Here's how the part is built. I have some questions about the finished solid (model axes, mm). Face numbers are marked on the shaded views. A direction names the side the tool comes from. Round coordinates to 2 decimals unless told otherwise and drop trailing zeros. Order: outer loops, then holes, each group sorted by start corner. A loop starts at its lowest first (then second) coordinate and runs counter-clockwise, first axis right, second up. Notation, with made-up numbers: M -8.75,77.5 L -4.75,77.5 A26 cw -4.75,112.5 Z; hole C -17.5,56 d1. An arc over 180 degrees is marked long. Write item = value, one per line. Start each with the question number.
Item 1: I want a section at B-B, the plane y = 0. List the corners of the cut face in (x, z) for me.
Item 2: For the marked faces 1, 2 and 3, which set-ups out of +Z, -Z, +X, -X, +Y, -Y let a thin tool reach every point of the face, with its end or its side?
Item 3: I'm going to push flat-ended pins straight in: P1, Ø6, axis at y = 14.5, z = 5, coming from the +X side; P2, Ø2, axis at x = -2, z = 4.5, coming from the +Y side; P3, Ø1, axis at x = -13, y = -31.5, coming from the -Z side. Where does each tip first touch, or does it pass through?
Item 4: Please list where these lines run through material, in increasing order: L1, parallel to Z at x = 10, y = 11; L2, parallel to Y at x = -7.5, z = 3.5; L3, parallel to Y at x = 0, z = -1.6.
Item 5: I want a section at A-A, the plane x = 0. List the corners of the cut face in (y, z) for me.
Item 6: We'd pull the mould along X, two halves only. Please class the marked faces 4, 5 and 6: pulls with the +X half, pulls with the -X half, needs draft (parallel to the pull), parting line crosses it, or undercut.
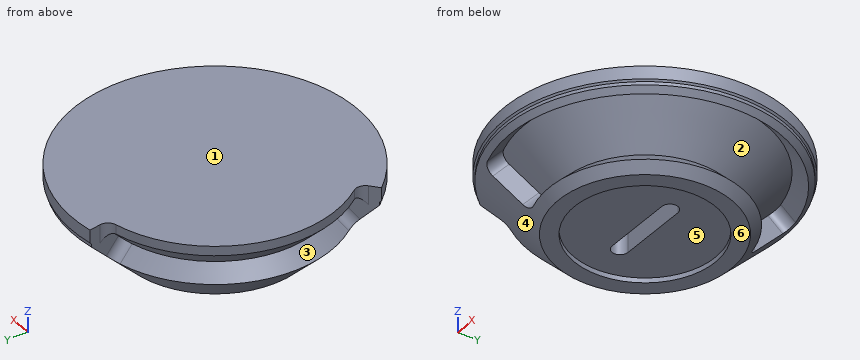
```python
from build123d import *

# Parameters (mm, degrees)
F3_W           = 8.3933982822
F3_H           = 16.3933982822
F4_ANGLE_BACK  = 40
F4_ANGLE       = 122
F6_ANGLE_START = 98
F6_ANGLE       = 196
F7_ANGLE_BACK  = 40
F7_ANGLE       = 122
F8_R           = 3
F8_2_R         = 3
F9_R           = 3
F13_DEPTH      = 10
F14_R          = 22
F15_DEPTH      = 1.5


with BuildPart() as f1:
    # F0 (on Front) → F1 (revolve)
    with BuildSketch(Plane.XZ):
        Polygon((-43.5, 14.5), (-27, -2), (0, -2), (0, 20), (-44, 20), (-44, 16), (-43.5, 15.5), align=None)
    revolve(axis=Axis((0, 0, 9.4880101401), (0, 0, -1)))


with BuildPart() as f4:
    # F3 (on Front) → F4 (revolve)
    with BuildSketch(Plane.XZ, mode=Mode.PRIVATE) as f4_sk:
        with Locations((-41.8033008589, 16.8033008589)):
            Rectangle(F3_W, F3_H)
    revolve(f4_sk.sketch.rotate(Axis((0, 0, 9.4880101401), (0, 0, -1)), -F4_ANGLE_BACK), axis=Axis((0, 0, 9.4880101401), (0, 0, -1)), revolution_arc=F4_ANGLE)

    # F8#2
    f8_2_edges = [f4.edges().sort_by_distance(p)[0] for p in [
        (-5.233827, 37.240617, 16.803301),
        (-28.808328, -24.173058, 16.803301),
    ]]
    fillet(f8_2_edges, radius=F8_2_R)


with BuildPart() as f6:
    # F5 (on Front) → F6 (revolve)
    with BuildSketch(Plane.XZ, mode=Mode.PRIVATE) as f6_sk:
        Polygon((-36.8994949366, -6.2426406871), (-25.5857864376, 5.0710678119), (-37.6066017178, 17.091883092), (-48.9203102168, 5.7781745931), align=None)
    revolve(f6_sk.sketch.rotate(Axis((0, 0, 9), (0, 0, -1)), F6_ANGLE_START), axis=Axis((0, 0, 9), (0, 0, -1)), revolution_arc=F6_ANGLE)

    # F9
    f9_edges = [f6.edges().sort_by_distance(p)[0] for p in [
        (4.348135, 30.938589, -0.585786),
        (6.021109, 42.842419, 11.435029),
        (-17.596833, -39.523134, 11.435029),
        (-12.707527, -28.541572, -0.585786),
    ]]
    fillet(f9_edges, radius=F9_R)


with BuildPart() as f7:
    # F2 (on Front) → F7 (revolve)
    with BuildSketch(Plane.XZ, mode=Mode.PRIVATE) as f7_sk:
        Polygon((-41.2877159425, 2.0970603683), (-31.9497474683, 11.4350288425), (-37.6066017178, 17.091883092), (-46.944570192, 7.7539146178), align=None)
    revolve(f7_sk.sketch.rotate(Axis((0, 0, 9), (0, 0, -1)), -F7_ANGLE_BACK), axis=Axis((0, 0, 9), (0, 0, -1)), revolution_arc=F7_ANGLE)

    # F8
    f8_edges = [f7.edges().sort_by_distance(p)[0] for p in [
        (-28.051576, -23.538067, 6.766045),
        (-5.096342, 36.262361, 6.766045),
    ]]
    fillet(f8_edges, radius=F8_R)


with BuildPart() as f1_1:
    add(f1.part)

    # F10: cut F7, F4, F6
    add(f7.part, mode=Mode.SUBTRACT)
    add(f4.part, mode=Mode.SUBTRACT)
    add(f6.part, mode=Mode.SUBTRACT)

    # F12 (on offset) → F13 (cut)
    with BuildSketch(Plane(origin=(0, 0, -2), x_dir=(1, 0, 0), z_dir=(0, 0, -1))):
        with BuildLine():
            ThreePointArc((-11, 2.5), (-13.5, 0), (-11, -2.5))
            Line((-11, -2.5), (0, -2.5))
            Line((0, -2.5), (11, -2.5))
            ThreePointArc((11, -2.5), (13.5, 0), (11, 2.5))
            Line((11, 2.5), (0, 2.5))
            Line((0, 2.5), (-11, 2.5))
        make_face()
    extrude(amount=-F13_DEPTH, mode=Mode.SUBTRACT)

    # F14 (on offset) → F15 (cut)
    with BuildSketch(Plane(origin=(0, 0, -2), x_dir=(1, 0, 0), z_dir=(0, 0, -1))):
        Circle(F14_R)
    extrude(amount=-F15_DEPTH, mode=Mode.SUBTRACT)


solid = f1_1.part
```
Filled in:
q1.outline = M -37.61,17.09 L -31.95,11.44 L -36.19,7.19 L -27,-2 L -22,-2 L -22,-0.5 L -13.5,-0.5 L -13.5,8 L 13.5,8 L 13.5,-0.5 L 22,-0.5 L 22,-2 L 27,-2 L 29.83,0.83 L 25.59,5.07 L 37.61,17.09 L 41.85,12.85 L 43.5,14.5 L 43.5,15.5 L 44,16 L 44,20 L -37.61,20 Z
q2.face_1 = +Z, +X, -X, +Y, -Y
q2.face_2 = none
q2.face_3 = -X
q3.P1 = 25.1
q3.P2 = 34.44
q3.P3 = 13.06
q4.L1 = -0.5 to 20
q4.L2 = -26.1 to -2.5, 2.5 to 31.62
q4.L3 = -27.4 to -22, 22 to 27.4
q5.outline = M -44,16 L -43.5,15.5 L -43.5,14.5 L -41.85,12.85 L -37.61,17.09 L -25.59,5.07 L -29.83,0.83 L -27,-2 L -22,-2 L -22,-0.5 L -2.5,-0.5 L -2.5,8 L 2.5,8 L 2.5,-0.5 L 22,-0.5 L 22,-2 L 27,-2 L 43.5,14.5 L 43.5,15.5 L 44,16 L 44,20 L -44,20 Z
q6.face_4 = parting line crosses it
q6.face_5 = undercut
q6.face_6 = needs draft
